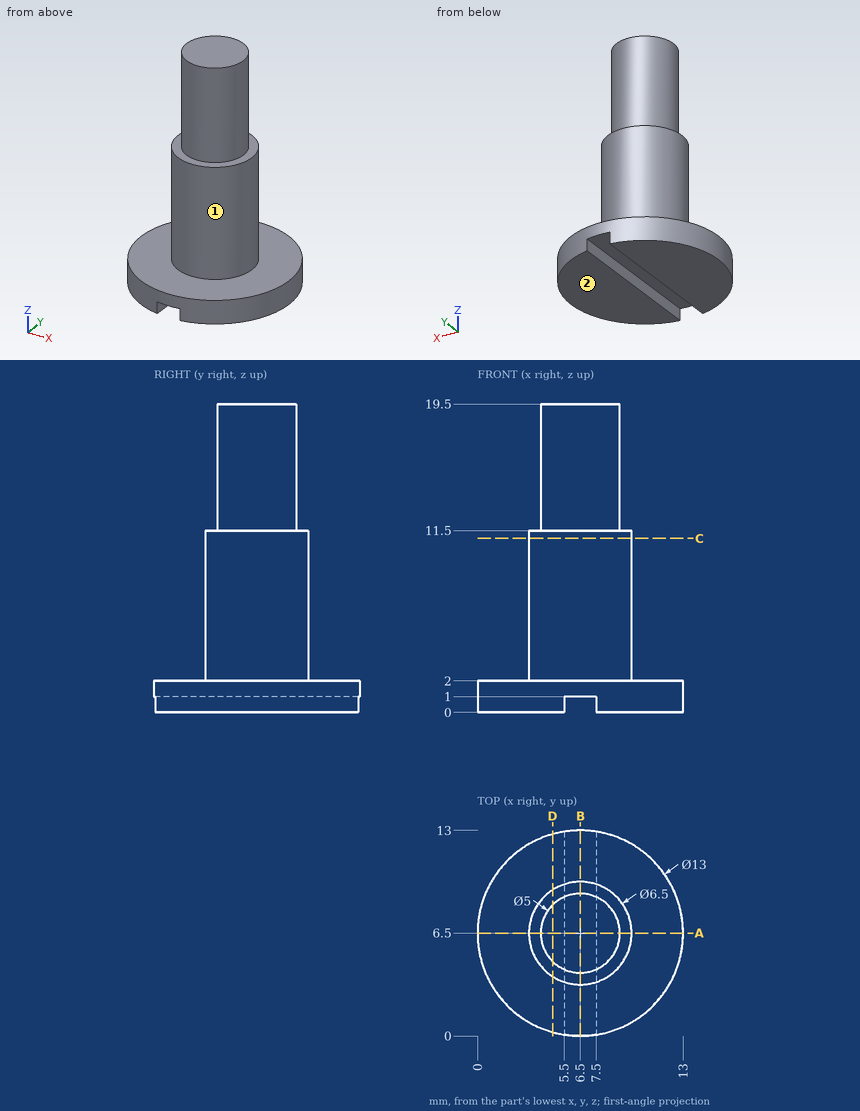
Print and shaded views of the part. All mm, measured from the part's lowest x, y and z. A direction names the side the tool comes from. Give positions to 0.01 mm unless a question says otherwise; leave off trailing zeros. Order: outer loops, then holes, each group sorted by start corner. A loop starts at its lowest first (then second) coordinate and runs counter-clockwise, first axis right, second up. Notation, with made-up numbers: M 27,83.25 L 62,83.25 A29 cw 62,109.25 Z; hole C 17.5,41.25 d1. An arc over 180 degrees is marked long. Use one line per item in the form item = value.
Q1. Wall check: probe 1 along Z at (x, y) = (6.5, 11); probe 2 along Z at (x, y) = (0.5, 4.25); probe 3 along Y at (x, z) = (3.5, 9). Give the ranges that are in metal, low to high.
Conclusion:
probe_1 = 1 to 2
probe_2 = 0 to 2
probe_3 = 5.25 to 7.75
Q2. Slice it at B-B, the plane x = 6.5. Write the cut outline in (y, z).
Conclusion:
outline = M 0,1 L 13,1 L 13,2 L 9.75,2 L 9.75,11.5 L 9,11.5 L 9,19.5 L 4,19.5 L 4,11.5 L 3.25,11.5 L 3.25,2 L 0,2 Z
Q3. Pin check, flat tips, straight feed: P1, Ø1, axis at x = 7.5, z = 9, coming from the -Y side; P2, Ø5, axis at x = 2.5, z = 7.5, coming from the -Y side; P3, Ø5, axis at x = 7, y = 10, coming from the +Z side; P4, Ø6, axis at y = 1.5, z = 5.5, coming from the +X side. Stop position of each tip, or through.
Conclusion:
P1 = 3.29
P2 = 3.62
P3 = 19.5
P4 = 9.06
Q4. Which spindle directions (+Z, -Z, +X, -X, +Y, -Y) get a long thin tool onto all of the face, cutting with end or side? Do the marked faces 1 and 2. Say none if no direction does.
Conclusion:
face_1 = +Z
face_2 = -Z, +X, -X, +Y, -Y
Q5. Slice it at A-A, the plane y = 6.5. Write the cut outline in (x, z).
Conclusion:
outline = M 0,0 L 5.5,0 L 5.5,1 L 7.5,1 L 7.5,0 L 13,0 L 13,2 L 9.75,2 L 9.75,11.5 L 9,11.5 L 9,19.5 L 4,19.5 L 4,11.5 L 3.25,11.5 L 3.25,2 L 0,2 Z
Q6. Slice it at C-C, the plane z = 11. Write the cut outline in (x, y).
Conclusion:
outline = C 6.5,6.5 d6.5
Q7. Slice it at D-D, the plane x = 4.75. Write the cut outline in (y, z).
Conclusion:
outline = M 0.24,0 L 12.76,0 L 12.76,2 L 9.24,2 L 9.24,11.5 L 8.29,11.5 L 8.29,19.5 L 4.71,19.5 L 4.71,11.5 L 3.76,11.5 L 3.76,2 L 0.24,2 Z
